Build history of the part. All positions in model axes, mm. A direction names the side the tool comes from. Give positions to 0.01 mm unless a question says otherwise; leave off trailing zeros. Order: outer loops, then holes, each group sorted by start corner. A loop starts at its lowest first (then second) coordinate and runs counter-clockwise, first axis right, second up. Notation, with made-up numbers: (43.5, 35.25) -> (51.5, 35.25) arc R11 ccw to (51.5, 56.25) -> close; hole circle Ø11 at (0, -40). An arc over 180 degrees is marked (long way). Use a Markdown table: item, result. Add a question column.
```python
from build123d import *

# Parameters (mm, degrees)
CROQUIS2_R                   = 1.6
SALIENTE_EXTRUIR1_DEPTH      = 15
CORTAR_EXTRUIR1_REACH        = 52.06
REDONDEO1_R                  = 1
CORTAR_EXTRUIR_L_MINA1_DEPTH = 16


# Read off the part's stored shape, not the designer's step: Cortar-Extruir-Lámina1
with BuildPart() as part:
    # Croquis2 → Saliente-Extruir1 (new, symmetric)
    with BuildSketch(Plane(origin=(0, 0, 0), x_dir=(0, 0, -1), z_dir=(1, 0, 0))):
        with BuildLine():
            Line((0, 16), (-45, 16))
            Line((-45, 16), (-45, 14))
            Line((-45, 14), (-5, 14))
            Line((-5, 14), (-5, 10.5))
            Line((-5, 10.5), (-33, 10.5))
            Line((-33, 10.5), (-33, 0))
            Line((-33, 0), (0, 0))
            Line((0, 0), (2, 2))
            Line((2, 2), (2, 2.75))
            Line((2, 2.75), (3, 3.75))
            Line((3, 3.75), (3.55, 3.75))
            ThreePointArc((3.55, 3.75), (4.578743846, 3.643024228), (5.563467425, 3.32667444))
            ThreePointArc((5.563467425, 3.32667444), (8.065241178, 2.700421444), (10.55, 3.391101056))
            Line((10.55, 3.391101056), (10.55, 12.108898944))
            ThreePointArc((10.55, 12.108898944), (8.065241178, 12.799578556), (5.563467425, 12.17332556))
            ThreePointArc((5.563467425, 12.17332556), (4.578743846, 11.856975772), (3.55, 11.75))
            Line((3.55, 11.75), (3, 11.75))
            Line((3, 11.75), (2, 12.75))
            Line((2, 12.75), (2, 14))
            Line((2, 14), (0, 16))
        make_face()
        with Locations((8, 7.75)):
            Circle(CROQUIS2_R, mode=Mode.SUBTRACT)
    extrude(amount=SALIENTE_EXTRUIR1_DEPTH, both=True)

    # Croquis3 → Cortar-Extruir1 (cut, up to next)
    with BuildSketch(Plane(origin=(0, 0, 0), x_dir=(1, 0, 0), z_dir=(0, 1, 0)), mode=Mode.PRIVATE) as cortar_extruir1_sk1:
        Polygon((11.6, -5), (-11.6, -5), (-11.6, -9), (-12.6, -9), (-12.6, -30.1), (-11.93, -30.1), (-12.6, -33), (12.6, -33), (11.93, -30.1), (12.6, -30.1), (12.6, -9), (11.6, -9), align=None)
    cortar_extruir1_tool1 = extrude(cortar_extruir1_sk1.sketch, amount=CORTAR_EXTRUIR1_REACH, mode=Mode.PRIVATE) & part.part
    add(cortar_extruir1_tool1.solids().sort_by_distance((0, 0, 19.104296))[0], mode=Mode.SUBTRACT)

    # Redondeo1
    redondeo1_edges = [part.edges().sort_by_distance(p)[0] for p in [
        (-15, 5.25, 33),
        (-15, 15, 45),
        (15, 15, 45),
        (15, 5.25, 33),
    ]]
    fillet(redondeo1_edges, radius=REDONDEO1_R)

    # Cortar-Extruir-Lámina1 outline → Cortar-Extruir-Lámina1 (cut)
    with BuildSketch(Plane(origin=(0, 0, 0), x_dir=(1, 0, 0), z_dir=(0, 1, 0))):
        Polygon((-15, 0), (-13, 2), (-8.9, 2), (-7.9, 3), (-7.9, 10.55), (-15, 10.55), align=None)
        Polygon((7.9, 3), (8.9, 2), (13, 2), (15, 0), (15, 10.55), (7.9, 10.55), align=None)
    extrude(amount=CORTAR_EXTRUIR_L_MINA1_DEPTH, mode=Mode.SUBTRACT)


solid = part.part
```
(1) Tool access for faces 4 (the face through (-11.6, 5, 7)), 5 (the face through (0.11, 11.86, -4.59)), 6 (the face through (12.6, 5, 20)): list every direction of +Z, -Z, +X, -X, +Y, -Y with a clear straight run to the whole face (end or side of a thin tool).
(2) Mould opens along Z. For faces 1 (the face through (-1, 0, 4)), 2 (the face through (12, 5, 9)), 3 (the face through (14.715, 5.176, 32.699)) say: released by +Z, released by -Z, zero draft, split by the parting line, or undercut.
(3) Band-saw the part on D-D on z = -8. Give the cut face in (x, y).
(4) Pin check, flat tips, straight feed: pin 1 Ø0.7 at (x, y) = (-12.5, 6) entering from -Z; pin 2 Ø1.1 at (x, y) = (13.5, 3) entering from +Z; pin 3 Ø6 at (x, y) = (-5.5, 3.5) entering from +Z. Stop position of each tip, or through.
(5) Band-saw the part on A-A on z = 18. Give the cut face in (x, y), plus the area to 3 significant figures.
(6) Wall check: probe 1 along Y at (x, z) = (1, -8); probe 2 along X at (y, z) = (7, 13); probe 3 along Z at (x, y) = (2.5, 7.75). Give the ranges that are in metal, low to high.
(7) Band-saw the part on C-C on x = -2.5. Give the cut face in (y, z).
Response:
| question | item | result |
|---|---|---|
| 1 | face 4 | +Z, -Y |
| 1 | face 5 | +X, -X, +Y |
| 1 | face 6 | -Y |
| 2 | face 1 | zero draft |
| 2 | face 2 | undercut |
| 2 | face 3 | released by +Z |
| 3 | outline | (-7.9, 2.7) -> (7.9, 2.7) -> (7.9, 6.15) -> (-7.9, 6.15) -> close; (-7.9, 9.35) -> (7.9, 9.35) -> (7.9, 12.8) -> (-7.9, 12.8) -> close |
| 4 | pin 1 | stops at z = -2 |
| 4 | pin 2 | stops at z = 33 |
| 4 | pin 3 | stops at z = 5 |
| 5 | outline | (-15, 0) -> (-12.6, 0) -> (-12.6, 10.5) -> (-15, 10.5) -> close; (-15, 14) -> (15, 14) -> (15, 16) -> (-15, 16) -> close; (12.6, 0) -> (15, 0) -> (15, 10.5) -> (12.6, 10.5) -> close |
| 5 | area | 110 mm² |
| 6 | probe 1 | y = 2.7 to 6.15, 9.35 to 12.8 |
| 6 | probe 2 | x = -15 to -12.6, 12.6 to 15 |
| 6 | probe 3 | z = -10.55 to -9.6, -6.4 to 5 |
| 7 | outline | (0, 0) -> (2, -2) -> (2.75, -2) -> (3.75, -3) -> (3.75, -3.55) arc R5 cw to (3.33, -5.56) arc R5.05 ccw to (3.39, -10.55) -> (12.11, -10.55) arc R5.05 ccw to (12.17, -5.56) arc R5 cw to (11.75, -3.55) -> (11.75, -3) -> (12.75, -2) -> (14, -2) -> (16, 0) -> (16, 45) -> (14, 45) -> (14, 5) -> (0, 5) -> close; hole circle Ø3.2 at (7.75, -8) |
